Geometry: see drawing. Coordinates: mm, zero at the bounding-box minimum. Round coordinates to 2 decimals unless told otherwise and drop trailing zeros. Order: outer loops, then holes, each group sorted by start corner. A loop starts at its lowest first (then second) coordinate and runs counter-clockwise, first axis right, second up.
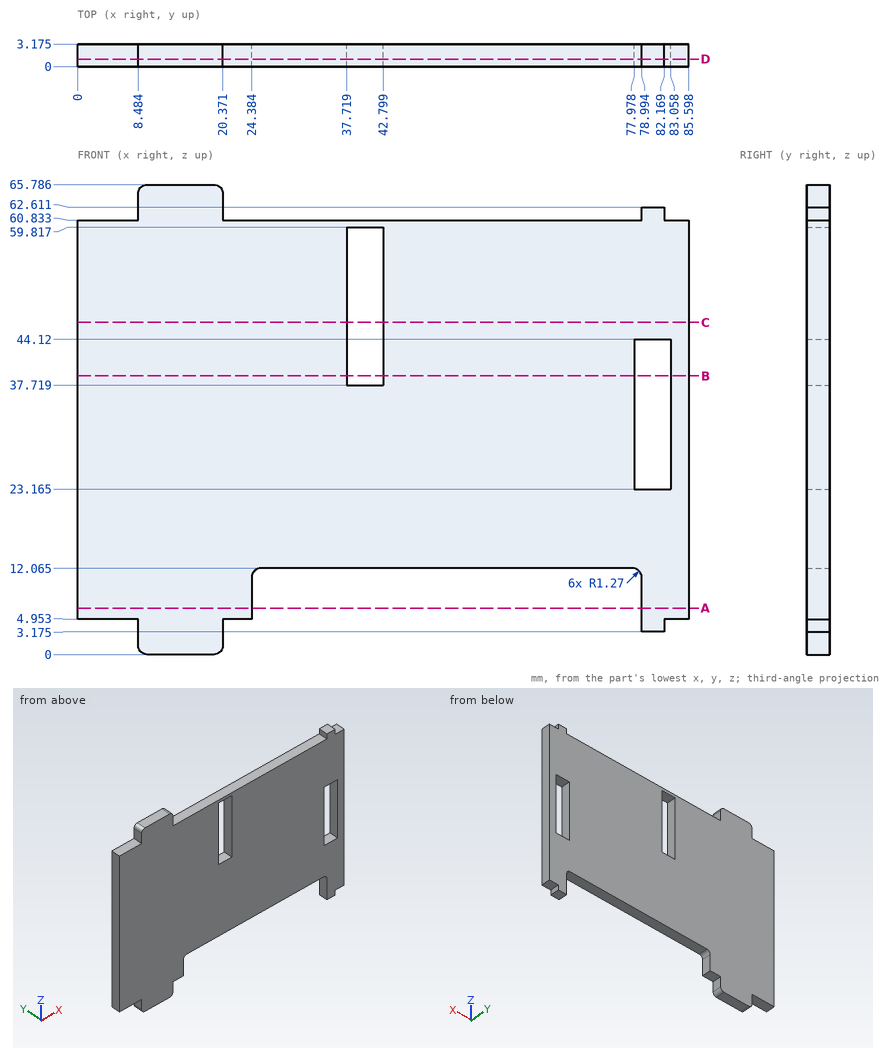
1. First-contact query: pin 1 (2 mm diameter, centred on x = 18.5, z = 55, fed in from -Y); pin 2 (1 mm diameter, centred on x = 44.5, y = 2, fed in from +Z); pin 3 (1 mm diameter, centred on y = 1.5, z = 62, fed in from -X); pin 4 (1.6 mm diameter, centred on x = 41.5, y = 2.5, fed in from -Z) (3 decimals). Flat tips, straight axial feed; report the tip coordinate or a pass-through.
2. Line query: line 1 along X through (y, z) = (0.3, 7.5); line 2 along X through (y, z) = (1.45, 4.5); line 3 along Z through (x, y) = (75.5, 2.85) (1 decimal). Output: solid intervals per line, ascending.
3. Section C-C on z = 46.5. Return loops of the section in (x, y) (1 decimal), plus the area to 3 significant figures.
4. Section B-B on z = 39. Return loops of the section in (x, y) (1 decimal).
5. Section D-D on y = 1.05. State how many separate pieces and enclosed holes the cut face has, plus the area to 3 significant figures.
6. Section A-A on z = 6.5. Return loops of the section in (x, y) (1 decimal).
Result:
1. pin 1: stops at y = 0
1. pin 2: stops at z = 60.83
1. pin 3: stops at x = 8.48
1. pin 4: stops at z = 12.065
2. line 1: x = 0 to 24.38, 78.99 to 85.6
2. line 2: x = 8.48 to 20.37, 78.99 to 82.17
2. line 3: z = 12.1 to 60.8
3. outline: (0, 0) - (37.7, 0) - (37.7, 3.2) - (0, 3.2) - close; (42.8, 0) - (85.6, 0) - (85.6, 3.2) - (42.8, 3.2) - close
3. area: 256 mm2
4. outline: (0, 0) - (37.7, 0) - (37.7, 3.2) - (0, 3.2) - close; (42.8, 0) - (78, 0) - (78, 3.2) - (42.8, 3.2) - close; (83.1, 0) - (85.6, 0) - (85.6, 3.2) - (83.1, 3.2) - close
5. separate pieces: 1
5. enclosed holes: 2
5. area: 4,300 mm2
6. outline: (0, 0) - (24.4, 0) - (24.4, 3.2) - (0, 3.2) - close; (79, 0) - (85.6, 0) - (85.6, 3.2) - (79, 3.2) - close
